Geometry: final body of the model. Coordinates: model frame, mm. Face numbers are marked on the shaded views. A direction names the side the tool comes from. Round coordinates to 2 decimals unless told otherwise and drop trailing zeros. Order: outer loops, then holes, each group sorted by start corner. A loop starts at its lowest first (then second) coordinate and runs counter-clockwise, first axis right, second up. Notation, with made-up numbers: (-21, 71) - (38, 71) arc R20 cw to (38, 88) - close; hole circle Ø1 at (24.5, 16). An arc over 180 degrees is marked (long way). Put each result on its own line as item: value. Start each with the question number.
(1) Access query for the marked faces 4, 5 and 6. Directions: +Z, -Z, +X, -X, +Y, -Y. A direction counts if a zero-diameter tool reaches every point of the face in a straight line with its end or side. Return the directions, or none.
(2) Pin query (flat end, axial travel): P1, Ø4, axis at x = 44, y = 68.5, coming from the -Z side; P2, Ø1.4, axis at y = 43.5, z = 2, coming from the +X side; P3, Ø3, axis at y = 37.5, z = 2, coming from the +X side; P4, Ø1.8, axis at y = 70.5, z = 2.5, coming from the +X side. Return the tip coordinate at first contact, or that it passes through.
(3) Section D-D (x = 37.5). Output: boundary loops of the cut face in (y, z).
(4) Section A-A (x = 89.5). Output: boundary loops of the cut face in (y, z).
(5) Section C-C (y = 74.5). Output: boundary loops of the cut face in (x, z), and give its area (3 significant figures).
(6) Material intervals for L1, parallel to Y at x = 42.5, z = 4.9; L2, parallel to Y at x = 83.5, z = 5.4; L3, parallel to Y at x = 34.5, z = 4.8, sorted ascending. Write a range as [from, to].
(7) Pull-direction query (Y, two-part tool) for the marked faces 1, 2 and 3; classes: released by +Y, released by -Y, zero draft, split by the parting line, or undercut.
(8) Section B-B (z = 3.45). Output: boundary loops of the cut face in (x, y), and give its area (3 significant figures).
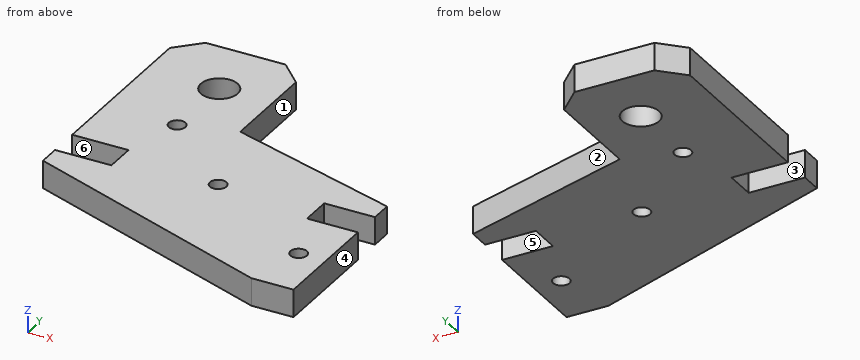
from build123d import *

# Parameters (mm, degrees)
MODEL_R                  = 1.8
MODEL_R_2                = 4
RESSALTO_EXTRUS_O1_DEPTH = 6


with BuildPart() as part:
    # Model → Ressalto-extrusão1 (new body)
    with BuildSketch(Plane.XY):
        Polygon((39.338603549, 33.894434028), (39.338603549, 40.60903008), (27.115699134, 40.60903008), (27.115699127, 78.895034597), (32.12692686, 83.90626233), (49.461276894, 83.906262358), (54.472504627, 78.895034645), (54.472504634, 57.076803542), (92.787264171, 45.319808703), (92.787264171, 40.60903008), (81.764808786, 40.60903008), (81.764808786, 33.894434028), (92.79400105, 33.894434035), (92.79400105, 8.643266236), (83.673566577, 8.643266228), (27.115699134, 29.183655407), (27.115699134, 33.894434028), align=None)
        with Locations((86.880751581, 21.371784671)):
            Circle(MODEL_R, mode=Mode.SUBTRACT)
        with Locations((60.638601845, 37.251732042)):
            Circle(MODEL_R, mode=Mode.SUBTRACT)
        with Locations((42.712190227, 53.576442757)):
            Circle(MODEL_R, mode=Mode.SUBTRACT)
        with Locations((42.946680849, 69.67437556)):
            Circle(MODEL_R_2, mode=Mode.SUBTRACT)
    extrude(amount=RESSALTO_EXTRUS_O1_DEPTH)


solid = part.part
Checks:
1. face 4: +Z, -Z, +X, +Y, -Y
1. face 5: +Z, -Z, +X
1. face 6: +Z, -Z, -X
2. P1: passes through
2. P2: stops at x = 92.79
2. P3: stops at x = 81.76
2. P4: stops at x = 54.47
3. outline: (25.41, 0) - (33.89, 0) - (33.89, 6) - (25.41, 6) - close; (40.61, 0) - (83.91, 0) - (83.91, 6) - (40.61, 6) - close
4. outline: (8.64, 0) - (33.89, 0) - (33.89, 6) - (8.64, 6) - close; (40.61, 0) - (46.33, 0) - (46.33, 6) - (40.61, 6) - close
5. outline: (27.12, 0) - (54.47, 0) - (54.47, 6) - (27.12, 6) - close
5. area: 164 mm²
6. L1: y = [23.6, 51.79], [55.36, 65.7], [73.65, 83.91]
6. L2: y = [8.71, 33.89], [40.61, 48.17]
6. L3: y = [26.5, 33.89], [40.61, 83.91]
7. face 1: zero draft
7. face 2: released by +Y
7. face 3: undercut
8. outline: (27.12, 29.18) - (83.67, 8.64) - (92.79, 8.64) - (92.79, 33.89) - (81.76, 33.89) - (81.76, 40.61) - (92.79, 40.61) - (92.79, 45.32) - (54.47, 57.08) - (54.47, 78.9) - (49.46, 83.91) - (32.13, 83.91) - (27.12, 78.9) - (27.12, 40.61) - (39.34, 40.61) - (39.34, 33.89) - (27.12, 33.89) - close; hole circle Ø8 at (42.95, 69.67); hole circle Ø3.6 at (42.71, 53.58); hole circle Ø3.6 at (60.64, 37.25); hole circle Ø3.6 at (86.88, 21.37)
8. area: 2,850 mm²
